```python
from build123d import *

# Parameters (mm, degrees)
PAD_DEPTH     = 6.3
THICKNESS_T   = -0.8
SKETCH001_W   = 2.8
SKETCH001_H   = 5.6
SKETCH001_W_2 = 1.2
SKETCH001_H_2 = 4
PAD001_DEPTH  = 9


with BuildPart() as part:
    # Sketch → Pad (new body, symmetric)
    with BuildSketch(Plane.YZ):
        with BuildLine():
            Line((-5.1, 0), (-5.1, 3.2))
            ThreePointArc((-5.1, 3.2), (-3.317216, 7.552005), (-2.6, 12.2))
            Line((-2.6, 12.2), (-0.5, 12.2))
            Line((-0.5, 12.2), (-0.5, 11.95))
            Line((-0.5, 11.95), (0.5, 11.95))
            Line((0.5, 11.95), (0.5, 12.2))
            Line((0.5, 12.2), (2.6, 12.2))
            ThreePointArc((2.6, 12.2), (3.317216, 7.552005), (5.1, 3.2))
            Line((5.1, 0), (5.1, 3.2))
            Line((-5.1, 0), (5.1, 0))
        make_face()
    extrude(amount=PAD_DEPTH, both=True)

    # Thickness
    thickness_openings = [part.faces().sort_by_distance(p)[0] for p in [
        (0, 0, 0),
    ]]
    offset(amount=THICKNESS_T, openings=thickness_openings)

    # Sketch001 → Pad001 (join)
    with BuildSketch(Plane.XY.offset(9)):
        Rectangle(SKETCH001_W, SKETCH001_H)
        Rectangle(SKETCH001_W_2, SKETCH001_H_2, mode=Mode.SUBTRACT)
    extrude(amount=-PAD001_DEPTH)


solid = part.part
```
Check sheet for the modelled part. Datum: model origin and axes. Units: mm. A direction names the side the tool comes from. Give positions to 0.01 mm unless a question says otherwise; leave off trailing zeros. Order: outer loops, then holes, each group sorted by start corner. A loop starts at its lowest first (then second) coordinate and runs counter-clockwise, first axis right, second up. Notation, with made-up numbers: M 29.5,5.5 L 34.5,5.5 A26 ccw 34.5,21.5 Z; hole C -31.5,64 d5. An arc over 180 degrees is marked long. Answer in a Markdown table with one row per item. Add a question column.
Q1. Sectioned sample at A-A, the plane z = 4.75. Record the boundary of the cut face in (x, y).
Q2. Gauge pin test, flat ends, axial feed: pin 1 Ø1.3 at (x, z) = (0, 6) entering from -Y; pin 2 Ø3 at (x, z) = (5, 10) entering from +Y; pin 3 Ø0.8 at (x, y) = (0, 0) entering from +Z. Record the tip position at first contact, or that the pin passes through.
Q3. Access from +Z, -Z, +X, -X, +Y, -Y to the whole of each face (thin tool, end or side, straight path). Record for faces 1 (the cylindrical face through (0.088, -3.335, 7.488)), 2 (the flat face through (1.4, 0, 5)).
Q4. Thickness scan on L1, parallel to X at y = 0.5, z = 7.75; L2, parallel to X at y = -2.25, z = 6; L3, parallel to Y at x = -2.5, z = 1. Record the ranges inside material, lowest first.
Q5. Sectioned sample at D-D, the plane z = 9.5. Record the boundary of the cut face in (x, y).
Q6. Release check for a two-part mould opening along Z. For faces 3 (the flat face through (0, -2.8, 3)), 4 (the flat face through (1, 0, 9)), 5 (the flat face through (0, 0, 11.15)), 6 (the flat face through (0, -2, 12.2)) record: released by +Z, released by -Z, zero draft, split by the parting line, or undercut.
Q7. Sectioned sample at B-B, the plane y = 0. Record the boundary of the cut face in (x, z).
Verdict:
| question | item | result |
|---|---|---|
| 1 | outline | M -6.3,-4.33 L 6.3,-4.33 L 6.3,4.33 L -6.3,4.33 Z; M -1.4,-2.8 L 1.4,-2.8 L 1.4,2.8 L -1.4,2.8 Z; hole M -5.5,-3.45 L 5.5,-3.45 L 5.5,3.45 L -5.5,3.45 Z; hole M -0.6,-2 L 0.6,-2 L 0.6,2 L -0.6,2 Z |
| 2 | pin 1 | y = -4.07 |
| 2 | pin 2 | y = 3.08 |
| 2 | pin 3 | z = 11.95 |
| 3 | face 1 | +Z, +X, -X, -Y |
| 3 | face 2 | -Z |
| 4 | L1 | -6.3 to -5.5, -1.4 to -0.6, 0.6 to 1.4, 5.5 to 6.3 |
| 4 | L2 | -6.3 to -5.5, -1.4 to 1.4, 5.5 to 6.3 |
| 4 | L3 | -5.1 to -4.3, 4.3 to 5.1 |
| 5 | outline | M -6.3,-2.88 L 6.3,-2.88 L 6.3,2.88 L -6.3,2.88 Z; hole M -5.5,-2.07 L 5.5,-2.07 L 5.5,2.07 L -5.5,2.07 Z |
| 6 | face 3 | zero draft |
| 6 | face 4 | undercut |
| 6 | face 5 | undercut |
| 6 | face 6 | released by +Z |
| 7 | outline | M -6.3,0 L -5.5,0 L -5.5,11.15 L 5.5,11.15 L 5.5,0 L 6.3,0 L 6.3,11.95 L -6.3,11.95 Z; M -1.4,0 L -0.6,0 L -0.6,9 L -1.4,9 Z; M 0.6,0 L 1.4,0 L 1.4,9 L 0.6,9 Z |
